from build123d import *

# Parameters (mm, degrees)
AUFSATZ_LINEAR_AUSTRAGEN1_DEPTH = 4


with BuildPart() as part:
    # Skizze1 → Aufsatz-Linear austragen1 (new body)
    with BuildSketch(Plane.XY):
        with BuildLine():
            Line((0, 0), (52.98962309, 0))
            Line((52.98962309, 0), (86.279270691, 47.542543867))
            ThreePointArc((86.279270691, 47.542543867), (88, 53), (89.720729309, 47.542543867))
            Line((89.720729309, 47.542543867), (123.01037691, 0))
            Line((123.01037691, 0), (140, 0))
            Line((140, 0), (140, 90))
            ThreePointArc((140, 90), (132.67766953, 107.67766953), (115, 115))
            Line((115, 115), (41.856576941, 115))
            Line((41.856576941, 115), (0, 0))
        make_face()
    extrude(amount=AUFSATZ_LINEAR_AUSTRAGEN1_DEPTH)


solid = part.part
CAD build for the part. Positions are in the model's coordinates, mm. A direction names the side the tool comes from. Give positions to 0.01 mm unless a question says otherwise; leave off trailing zeros. Order: outer loops, then holes, each group sorted by start corner. A loop starts at its lowest first (then second) coordinate and runs counter-clockwise, first axis right, second up. Notation, with made-up numbers: (-1.75, 5) - (9.25, 5) arc R24 cw to (9.25, 15) - close; hole circle Ø6 at (85.5, 73). An arc over 180 degrees is marked (long way). Write each question's results on one line, items separated by ' | '.
1. Saw through at B-B on z = 3.25. List the corners of the cut face in (x, y).
Calculated:
outline: (0, 0) - (52.99, 0) - (86.28, 47.54) arc R3 cw (long way) to (89.72, 47.54) - (123.01, 0) - (140, 0) - (140, 90) arc R25 ccw to (115, 115) - (41.86, 115) - close
2. Saw through at A-A on y = 20. List the corners of the cut face in (x, z), and give its area (3 significant figures).
Calculated:
outline: (7.28, 0) - (66.99, 0) - (66.99, 4) - (7.28, 4) - close; (109.01, 0) - (140, 0) - (140, 4) - (109.01, 4) - close | area: 363 mm2
3. Probe L1, parallel to Y at x = 88, z = 3.1; L2, parallel to X at y = 50, z = 2.9; L3, parallel to X at y = 6, z = 1.75. List the from-to ranges inside material, lowest first. Write a range as from..to.
Calculated:
L1: y = 53..115 | L2: x = 18.2..85, 91..140 | L3: x = 2.18..57.19, 118.81..140
4. Pull direction X, two halves, no side cores. Call faces 1 (the face through (85, 58, 0)), 2 (the face through (21.22, 58.3, 1.97)), 3 (the face through (140, 44, 2)), 4 (the face through (106.133, 24.104, 1.972)): released by +X, released by -X, zero draft, split by the parting line, or undercut.
Calculated:
face 1: zero draft | face 2: released by -X | face 3: released by +X | face 4: undercut
5. 3-axis set-ups, long thin cutter, end or side, ignore diameter. For faces 5 (the face through (69.401, 23.438, 1.972)), 6 (the face through (131, 0, 2)): which of +Z, -Z, +X, -X, +Y, -Y reach the whole face in a straight line?
Calculated:
face 5: +Z, -Z, -Y | face 6: +Z, -Z, +X, -X, -Y
6. Saw through at C-C on x = 88. List the corners of the cut face in (y, z), and give its area (3 significant figures).
Calculated:
outline: (53, 0) - (115, 0) - (115, 4) - (53, 4) - close | area: 248 mm2
7. Pin check, flat tip, straight feed: pin 1 (2 mm diameter, centred on y = 51.5, z = 2.5, fed in from -X). Stop position of the tip, or through.
Calculated:
pin 1: stops at x = 18.38
8. Saw through at D-D on y = 50. List the corners of the cut face in (x, z), and give its area (3 significant figures).
Calculated:
outline: (18.2, 0) - (85, 0) - (85, 4) - (18.2, 4) - close; (91, 0) - (140, 0) - (140, 4) - (91, 4) - close | area: 463 mm2
